```python
from build123d import *

# Parameters (mm, degrees)
SKETCH1_W           = 25.4
SKETCH1_H           = 25.4
SKETCH1_W_2         = 19.05
SKETCH1_H_2         = 19.05
BOSS_EXTRUDE1_DEPTH = 863.6
CUT_EXTRUDE1_REACH  = 866.067
CUT_EXTRUDE2_REACH  = 866.067
SKETCH4_R           = 3.3782
CUT_EXTRUDE3_DEPTH  = 865.066785613
CUT_EXTRUDE4_REACH  = 866.067
SKETCH5_R           = 4.7625
SKETCH6_R           = 1.5875
CUT_EXTRUDE5_DEPTH  = 865.066785613


with BuildPart() as part:
    # Sketch1 → Boss-Extrude1 (new body)
    with BuildSketch(Plane(origin=(0, 0, 0), x_dir=(1, 0, 0), z_dir=(0, 1, 0))):
        Rectangle(SKETCH1_W, SKETCH1_H)
        Rectangle(SKETCH1_W_2, SKETCH1_H_2, mode=Mode.SUBTRACT)
    extrude(amount=BOSS_EXTRUDE1_DEPTH)

    # Sketch2 → Cut-Extrude1 (cut, up to next)
    with BuildSketch(Plane(origin=(0, 0, -12.7), x_dir=(-1, 0, 0), z_dir=(0, 0, -1)), mode=Mode.PRIVATE) as cut_extrude1_sk1:
        with BuildLine():
            Line((-3.175, 711.2), (-3.175, 825.5))
            ThreePointArc((-3.175, 825.5), (0, 828.675), (3.175, 825.5))
            Line((3.175, 825.5), (3.175, 711.2))
            ThreePointArc((3.175, 711.2), (0, 708.025), (-3.175, 711.2))
        make_face()
    cut_extrude1_tool1 = extrude(cut_extrude1_sk1.sketch, amount=-CUT_EXTRUDE1_REACH, mode=Mode.PRIVATE) & part.part
    add(cut_extrude1_tool1.solids().sort_by_distance((0, 768.35, -12.7))[0], mode=Mode.SUBTRACT)

    # Sketch3 → Cut-Extrude2 (cut, up to next)
    with BuildSketch(Plane.XY.offset(12.7), mode=Mode.PRIVATE) as cut_extrude2_sk1:
        with BuildLine():
            Line((3.175, 844.55), (3.175, 774.7))
            ThreePointArc((3.175, 774.7), (0, 771.525), (-3.175, 774.7))
            Line((-3.175, 774.7), (-3.175, 844.55))
            ThreePointArc((-3.175, 844.55), (0, 847.725), (3.175, 844.55))
        make_face()
    cut_extrude2_tool1 = extrude(cut_extrude2_sk1.sketch, amount=-CUT_EXTRUDE2_REACH, mode=Mode.PRIVATE) & part.part
    add(cut_extrude2_tool1.solids().sort_by_distance((0, 809.625, 12.7))[0], mode=Mode.SUBTRACT)

    # Sketch4 → Cut-Extrude3 (cut, through all)
    with BuildSketch(Plane.ZY.offset(12.7)):
        with Locations((-3.175, 793.75)):
            Circle(SKETCH4_R)
    extrude(amount=-CUT_EXTRUDE3_DEPTH, mode=Mode.SUBTRACT)

    # Sketch5 → Cut-Extrude4 (cut, up to next)
    with BuildSketch(Plane.ZY.offset(12.7), mode=Mode.PRIVATE) as cut_extrude4_sk1:
        with Locations((0, 854.075)):
            Circle(SKETCH5_R)
    cut_extrude4_tool1 = extrude(cut_extrude4_sk1.sketch, amount=-CUT_EXTRUDE4_REACH, mode=Mode.PRIVATE) & part.part
    # Sketch5 → Cut-Extrude4 (cut, up to next)
    with BuildSketch(Plane.ZY.offset(12.7), mode=Mode.PRIVATE) as cut_extrude4_sk2:
        with Locations((0, 835.025)):
            Circle(SKETCH5_R)
    cut_extrude4_tool2 = extrude(cut_extrude4_sk2.sketch, amount=-CUT_EXTRUDE4_REACH, mode=Mode.PRIVATE) & part.part
    add(cut_extrude4_tool1.solids().sort_by_distance((-12.7, 854.075, 0))[0], mode=Mode.SUBTRACT)
    add(cut_extrude4_tool2.solids().sort_by_distance((-12.7, 835.025, 0))[0], mode=Mode.SUBTRACT)

    # Sketch6 → Cut-Extrude5 (cut, through all)
    with BuildSketch(Plane.XY.offset(12.7)):
        with Locations((0, 19.05)):
            Circle(SKETCH6_R)
        with Locations((0, 38.1)):
            Circle(SKETCH6_R)
        with Locations((0, 57.15)):
            Circle(SKETCH6_R)
        with Locations((0, 76.2)):
            Circle(SKETCH6_R)
        with Locations((0, 95.25)):
            Circle(SKETCH6_R)
        with Locations((0, 114.3)):
            Circle(SKETCH6_R)
        with Locations((0, 133.35)):
            Circle(SKETCH6_R)
        with Locations((0, 152.4)):
            Circle(SKETCH6_R)
        with Locations((0, 171.45)):
            Circle(SKETCH6_R)
        with Locations((0, 190.5)):
            Circle(SKETCH6_R)
        with Locations((0, 209.55)):
            Circle(SKETCH6_R)
        with Locations((0, 228.6)):
            Circle(SKETCH6_R)
        with Locations((0, 247.65)):
            Circle(SKETCH6_R)
        with Locations((0, 266.7)):
            Circle(SKETCH6_R)
        with Locations((0, 285.75)):
            Circle(SKETCH6_R)
    extrude(amount=-CUT_EXTRUDE5_DEPTH, mode=Mode.SUBTRACT)


solid = part.part
```
Work out the finished part from the listing and answer in its coordinate system (mm). A direction names the side the tool comes from. Round coordinates to 2 decimals unless told otherwise and drop trailing zeros. Write each loop counter-clockwise with the first axis right and the second up, starting at its lowest first coordinate (ties: lowest second). Pieces come first, ordered by that corner, then holes. Notation, with made-up numbers: (35, 56.25) -> (55, 56.25) arc R30 ccw to (55, 87.25) -> close; hole circle Ø2 at (-28.5, 31). An arc over 180 degrees is marked (long way). Write each question's results on one line, items separated by ' | '.
1) Consider line 1 along Z through (x, y) = (1.25, 258) (3 decimals); line 2 along X through (y, z) = (190.5, 11.6). Determine where each line is inside the solid, lowest interval first. Write a range as [from, to].
Findings:
line 1: z = [-12.7, -9.525], [9.525, 12.7] | line 2: x = [-12.7, -1.59], [1.59, 12.7]
2) Which of the six approach directions +Z, -Z, +X, -X, +Y, -Y give full straight-line access (tool end or side, diameter ignored) to faces 4 (the flat face through (0, 426, -12.7)), 5 (the flat face through (9.525, 426, 0))?
Findings:
face 4: -Z, +X, -X, +Y, -Y | face 5: +Y, -Y
3) For a pull along X with two mould halves and no side action, classify faces 1 (the flat face through (11, 863.6, 0)), 2 (the flat face through (-12.7, 426, 0)), 3 (the flat face through (0, 426, -9.525)) as +X half, -X half, draft (parallel to the pull), parting line (faces both ways), or undercut.
Findings:
face 1: draft | face 2: -X half | face 3: undercut
4) The part is cut by section A-A (y = 517). Write down the section's boundary in (x, z) (3 decimals), and give its area (3 significant figures).
Findings:
outline: (-12.7, -12.7) -> (12.7, -12.7) -> (12.7, 12.7) -> (-12.7, 12.7) -> close; hole (-9.525, -9.525) -> (9.525, -9.525) -> (9.525, 9.525) -> (-9.525, 9.525) -> close | area: 282 mm²
